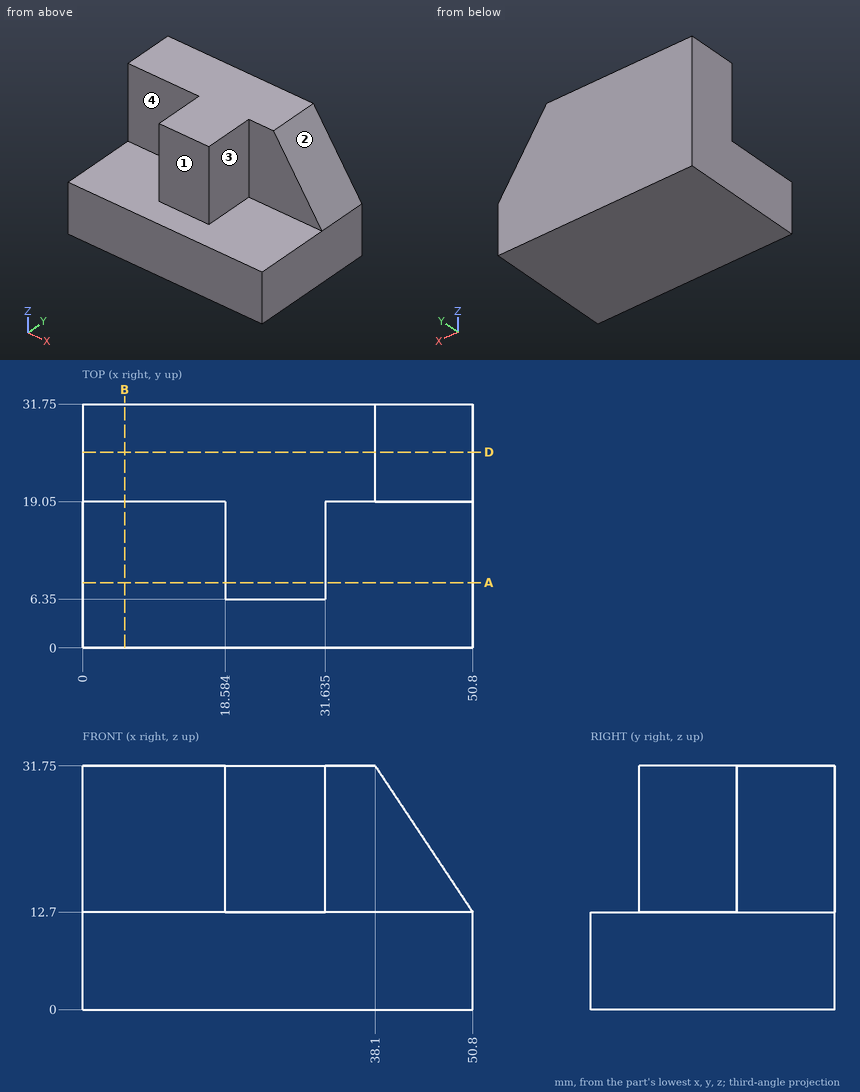
Source: three-view drawing plus pictorial views. Frame: mm from the lowest corner of the part. A direction names the side the tool comes from. Give positions to 0.01 mm unless a question says otherwise; leave off trailing zeros. Loops run counter-clockwise (first coordinate to the right, second up) from the corner with the lowest first, then second, coordinate; pieces in that order, holes last. Notation, with made-up numbers: (-7, -35.75) -> (1, -35.75) arc R35 ccw to (1, -1.75) -> close; hole circle Ø7 at (41, -12.5). An arc over 180 degrees is marked (long way). Use a Markdown table: item, result. Add a question column.
(1) Section query D-D (y = 25.5). Output: boundary loops of the cut face in (x, z), then the cut area to 3 significant figures.
(2) Access query for the marked faces 1, 2, 3 and 4. Directions: +Z, -Z, +X, -X, +Y, -Y. A direction counts if a zero-diameter tool reaches every point of the face in a straight line with its end or side. Return the directions, or none.
(3) Section query A-A (y = 8.5). Output: boundary loops of the cut face in (x, z) (3 decimals).
(4) First-contact query: pin 1 Ø6 at (x, y) = (38.5, 10.5) entering from +Z; pin 2 Ø12 at (x, z) = (44.5, 10) entering from -Y; pin 3 Ø15 at (x, z) = (11.5, 21) entering from -Y; pin 4 Ø1 at (y, z) = (12, 15.5) entering from +X (3 decimals). Flat tips, straight axial feed; report the tip coordinate or a pass-through.
(5) Ray query, line 1 (Z direction, x = 33, y = 2); line 2 (Y direction, x = 36, z = 22); line 3 (X direction, y = 8, z = 28) (3 decimals). Return the intervals inside material, ascending.
(6) Section query B-B (x = 5.5). Output: boundary loops of the cut face in (y, z).
Checked values:
| question | item | result |
|---|---|---|
| 1 | outline | (0, 0) -> (50.8, 0) -> (50.8, 12.7) -> (38.1, 31.75) -> (0, 31.75) -> close |
| 1 | area | 1,490 mm^2 |
| 2 | face 1 | +Z, +X, -X, -Y |
| 2 | face 2 | +Z, +X, +Y, -Y |
| 2 | face 3 | +Z, +X, -Y |
| 2 | face 4 | +Z, -X, -Y |
| 3 | outline | (0, 0) -> (50.8, 0) -> (50.8, 12.7) -> (31.635, 12.7) -> (31.635, 31.75) -> (18.584, 31.75) -> (18.584, 12.7) -> (0, 12.7) -> close |
| 4 | pin 1 | z = 12.7 |
| 4 | pin 2 | y = 0 |
| 4 | pin 3 | y = 6.35 |
| 4 | pin 4 | x = 31.635 |
| 5 | line 1 | 0 to 12.7 |
| 5 | line 2 | 19.05 to 31.75 |
| 5 | line 3 | 18.584 to 31.635 |
| 6 | outline | (0, 0) -> (31.75, 0) -> (31.75, 31.75) -> (19.05, 31.75) -> (19.05, 12.7) -> (0, 12.7) -> close |
